Part model, mm, in its own coordinate system. A direction names the side the tool comes from. Round coordinates to 2 decimals unless told otherwise and drop trailing zeros. Write each loop counter-clockwise with the first axis right and the second up, starting at its lowest first coordinate (ties: lowest second). Pieces come first, ordered by that corner, then holes. Notation, with made-up numbers: (87, 16) -> (142, 16) arc R15 cw to (142, 38) -> close; hole circle Ø8 at (66, 72.5). An arc over 180 degrees is marked (long way). Return JSON: item names as keys, results as strings. Group by question number.
(1) Tool access for faces 1 (the flat face through (0, 34.709, 1)), 2 (the flat face through (12.9, -15, 28)), 3 (the flat face through (0, 0, 3)): list every direction of +Z, -Z, +X, -X, +Y, -Y with a clear straight run to the whole face (end or side of a thin tool).
(2) Mould opens along X. For faces 4 (the flat face through (-22, -15, 52)), 5 (the cylindrical face through (-15, -14.8, 45.1)), 6 (the flat face through (23, -15, 51)) say: +X half, -X half, draft (parallel to the pull), parting line (faces both ways), or undercut.
(3) Saw through at D-D (x = 15). List the corners of the cut face in (y, z).
(4) Drill centre lines: L1, parallel to Y at x = 15.5, z = 1.25; L2, parallel to Y at x = 0, z = 1.85; L3, parallel to Y at x = 15.5, z = 1.5. Where is each one in solid material? Low to high. Write a range as from..to.
(5) Saw through at C-C (y = 20.5). List the corners of the cut face in (x, z).
(6) Saw through at B-B (z = 24.5). List the corners of the cut face in (x, y), plus the area to 3 significant figures.
(7) Saw through at A-A (x = 0). List the corners of the cut face in (y, z).
(8) Drop flat-ended pins along their axis: pin 1 Ø20 at (x, y) = (0, 11.71) entering from -Z; pin 2 Ø5.5 at (x, y) = (-15.5, -3.79) entering from +Z. Give the stop position or say it passes through.
from build123d import *

# Parameters (mm, degrees)
SKETCH_1_R          = 1.75
SKETCH_1_R_2        = 11.05
EXTRUDE_1_DEPTH     = 3
SKETCH_2_W          = 50
SKETCH_2_H          = 3
EXTRUDE_2_DEPTH     = 51
FILLET_1_R          = 2
CUT_EXTRUDE_1_DEPTH = 51
CHAMFER_1_SIZE      = 5


with BuildPart() as part:
    # 草图1 → 凸台-拉伸1 (new body)
    with BuildSketch(Plane.XY):
        Polygon((25, 29.708680022), (25, -16.291319978), (-25, -16.291319978), (-25, 29.708680022), (-20, 34.708680022), (20, 34.708680022), align=None)
        with Locations((-15.5, 27.208680022)):
            Circle(SKETCH_1_R, mode=Mode.SUBTRACT)
        with Locations((15.5, 27.208680022)):
            Circle(SKETCH_1_R, mode=Mode.SUBTRACT)
        with Locations((-15.5, -3.791319978)):
            Circle(SKETCH_1_R, mode=Mode.SUBTRACT)
        with Locations((15.5, -3.791319978)):
            Circle(SKETCH_1_R, mode=Mode.SUBTRACT)
        with Locations((0, 11.708680022)):
            Circle(SKETCH_1_R_2, mode=Mode.SUBTRACT)
    extrude(amount=EXTRUDE_1_DEPTH)

    # 草图2 → 凸台-拉伸2 (add)
    with BuildSketch(Plane.XY.offset(3)):
        with Locations((0, -14.791319978)):
            Rectangle(SKETCH_2_W, SKETCH_2_H)
    extrude(amount=EXTRUDE_2_DEPTH)

    # 圆角1
    fillet_1_edges = [part.edges().sort_by_distance(p)[0] for p in [
        (0, -16.291319978, 0),
    ]]
    fillet(fillet_1_edges, radius=FILLET_1_R)

    # 草图3 → 切除-拉伸1 (cut)
    with BuildSketch(Plane(origin=(0, -13.291319978, 0), x_dir=(1, 0, 0), z_dir=(0, 1, 0))):
        with BuildLine():
            Line((-17.1, -13), (-17.1, -43))
            ThreePointArc((-17.1, -43), (-15, -45.1), (-12.9, -43))
            Line((-12.9, -43), (-12.9, -13))
            ThreePointArc((-12.9, -13), (-15, -10.9), (-17.1, -13))
        make_face()
        with BuildLine():
            Line((12.9, -13), (12.9, -43))
            ThreePointArc((12.9, -43), (15, -45.1), (17.1, -43))
            Line((17.1, -43), (17.1, -13))
            ThreePointArc((17.1, -13), (15, -10.9), (12.9, -13))
        make_face()
    extrude(amount=-CUT_EXTRUDE_1_DEPTH, mode=Mode.SUBTRACT)

    # 倒角1
    chamfer_1_edges = [part.edges().sort_by_distance(p)[0] for p in [
        (-25, -14.791319978, 54),
        (25, -14.791319978, 54),
    ]]
    chamfer(chamfer_1_edges, length=CHAMFER_1_SIZE)


solid = part.part
Computed values:
{
 "1": {"face 1": "+Z, -Z, +X, -X, +Y", "face 2": "+Y, -Y", "face 3": "+Z, +X, -X, +Y"},
 "2": {"face 4": "-X half", "face 5": "undercut", "face 6": "+X half"},
 "3": {"outline": "(-16.29, 2) arc R2 ccw to (-14.29, 0) -> (-5.47, 0) -> (-5.47, 3) -> (-13.29, 3) -> (-13.29, 10.9) -> (-16.29, 10.9) -> close; (-16.29, 45.1) -> (-13.29, 45.1) -> (-13.29, 54) -> (-16.29, 54) -> close; (-2.11, 0) -> (25.53, 0) -> (25.53, 3) -> (-2.11, 3) -> close; (28.89, 0) -> (34.71, 0) -> (34.71, 3) -> (28.89, 3) -> close"},
 "4": {"L1": "-16.15..-5.54, -2.04..25.46, 28.96..34.71", "L2": "-16.29..0.66, 22.76..34.71", "L3": "-16.23..-5.54, -2.04..25.46, 28.96..34.71"},
 "5": {"outline": "(-25, 0) -> (-6.69, 0) -> (-6.69, 3) -> (-25, 3) -> close; (6.69, 0) -> (25, 0) -> (25, 3) -> (6.69, 3) -> close"},
 "6": {"outline": "(-25, -16.29) -> (-17.1, -16.29) -> (-17.1, -13.29) -> (-25, -13.29) -> close; (-12.9, -16.29) -> (12.9, -16.29) -> (12.9, -13.29) -> (-12.9, -13.29) -> close; (17.1, -16.29) -> (25, -16.29) -> (25, -13.29) -> (17.1, -13.29) -> close", "area": "125 mm2"},
 "7": {"outline": "(-16.29, 2) arc R2 ccw to (-14.29, 0) -> (0.66, 0) -> (0.66, 3) -> (-13.29, 3) -> (-13.29, 54) -> (-16.29, 54) -> close; (22.76, 0) -> (34.71, 0) -> (34.71, 3) -> (22.76, 3) -> close"},
 "8": {"pin 1": "through", "pin 2": "z = 3"}
}
